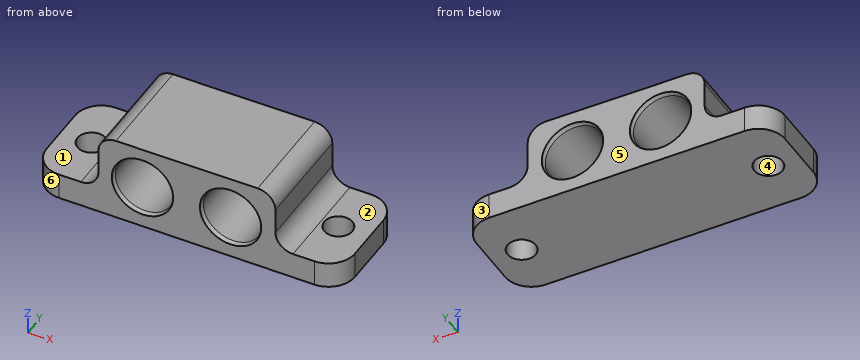
Autodesk Fusion 360 part; units mm, degrees
sketch "Sketch1" plane through (0, 0, 0) normal (0, 1, 0) x (1, 0, 0)
  circle A0 centre (-5, -5) radius 3.35
  circle A1 centre (5, -5) radius 3.35
  line L0 (-10, -5) -> (-10, -7.815)
  line L1 (-8.0118, -9.815) -> (8.0725, -9.9095)
  line L2 (10.0842, -7.9096) -> (10.0842, -5)
  line L3 (-17.5, 0) -> (17.5, 0)
  line L4 (17.5, 0) -> (17.5, -3)
  line L5 (-17.5, -3) -> (-17.5, 0)
  line L6 (-12, -3) -> (-17.5, -3)
  line L7 (17.5, -3) -> (12.0842, -3)
  arc A2 (-10, -7.815) -> (-8.0118, -9.815) centre (-8, -7.815) ccw
  arc A3 (-10, -5) -> (-12, -3) centre (-12, -5) ccw
  arc A4 (8.0725, -9.9095) -> (10.0842, -7.9096) centre (8.0842, -7.9096) ccw
  arc A5 (12.0842, -3) -> (10.0842, -5) centre (12.0842, -5) ccw
  point P0 (0, -5)
  dimension "d1" = 6.7
  dimension "d2" = 35
  dimension "d12" = 3
  dimension "d13" = 2
extrude "Extrude1" add sketch "Sketch1" along normal blind 12
sketch "Sketch2" plane through (0, 0, 0) normal (0, 0, -1) x (1, 0, 0)
  line L0 (17.5, 0) -> (-17.5, 0)
  line L1 (-17.5, 0) -> (-17.5, -12)
  line L2 (-17.5, -12) -> (17.5, -12)
  line L3 (17.5, -12) -> (17.5, 0)
  circle A0 centre (-14, -6) radius 1.6
  circle A1 centre (14, -6) radius 1.6
  dimension "d6" = 3.2
  dimension "d7" = 3.2
extrude "Extrude2" cut sketch "Sketch2" against normal blind 5 contours A0 | A1
fillet "Fillet1" radius 3 4 edges at (17.5, 0, 1.5) (17.5, 12, 1.5) (-17.5, 0, 1.5) (-17.5, 12, 1.5)
chamfer "Chamfer1" distance 0.5 angle 15 2 edges at (-8.1233, 0, 3.7886) (1.8767, 0, 3.7886) measured on face at (-1.6542, 8, 5.167) measured on face at (8.3458, 8, 5.167)
chamfer "Chamfer1" distance 0.5 angle 15 2 edges at (1.8767, 12, 3.7886) (-8.1233, 12, 3.7886) measured on face at (8.3458, 8, 5.167) measured on face at (-1.6542, 8, 5.167)
Could you check a few things on this model? Use its own coordinates, in mm. Face numbers are marked on the shaded views. A direction names the side the tool comes from. Coordinates: 2 decimals unless noted, no trailing zeros. Loops run counter-clockwise (first coordinate to the right, second up) from the corner with the lowest first, then second, coordinate; pieces in that order, holes last.
1) Which directions (+Z, -Z, +X, -X, +Y, -Y) give clear straight access to the entire face, cutting with the end or side of a thin tool? Please do the marked faces 1, 2 and 3.
Reported:
face 1: +Z, -X, +Y, -Y
face 2: +Z, +X, +Y, -Y
face 3: +Z, -Z, +X, +Y
2) Imagine slicing it at D-D (x = 5). List the corners of the cut face in (y, z) for me.
Reported:
outline: (0, 0) - (12, 0) - (12, 1.52) - (11.5, 1.65) - (0.5, 1.65) - (0, 1.52) - close; (0, 8.48) - (0.5, 8.35) - (11.5, 8.35) - (12, 8.48) - (12, 9.89) - (0, 9.89) - close
3) Thinking about a two-plate mould opening in X: for the marked faces 4, 5 and 6, which applies, released by +X, released by -X, zero draft, split by the parting line, or undercut?
Reported:
face 4: undercut
face 5: zero draft
face 6: released by -X
4) Imagine slicing it at A-A (x = -14). List the corners of the cut face in (y, z) for me, and give its area (3 significant figures).
Reported:
outline: (0, 0) - (4.4, 0) - (4.4, 3) - (0, 3) - close; (7.6, 0) - (12, 0) - (12, 3) - (7.6, 3) - close
area: 26.4 mm2
5) Imagine slicing it at B-B (y = 3.75). State how many separate pieces and enclosed holes the cut face has, and give its area (3 significant figures).
Reported:
separate pieces: 1
enclosed holes: 2
area: 172 mm2
6) Please list where these lines run through material, in increasing order: line 1 along X through (y, z) = (6, 1.2); line 2 along X through (y, z) = (6, 5); line 3 along Y through (x, z) = (-14, 1.65).
Reported:
line 1: x = -17.5 to -15.6, -12.4 to 12.4, 15.6 to 17.5
line 2: x = -10 to -8.35, -1.65 to 1.65, 8.35 to 10.08
line 3: y = 0 to 4.4, 7.6 to 12
7) Will these pins go through, and if not, where does the flat tip stop? pin 1 Ø1.5 at (y, z) = (6.5, 7) entering from +X; pin 2 Ø2 at (y, z) = (7, 8) entering from -X; pin 3 Ø1.9 at (x, y) = (-14, 6) entering from -Z; pin 4 Ø4.5 at (x, y) = (16, 8) entering from +Z.
Reported:
pin 1: stops at x = 10.08
pin 2: stops at x = -10
pin 3: passes through
pin 4: stops at z = 3
